Design review of the part built by this model. Coordinates are the model's own, in mm. Give positions to 0.01 mm unless a question says otherwise; leave off trailing zeros. Order: outer loops, then holes, each group sorted by start corner. A loop starts at its lowest first (then second) coordinate and runs counter-clockwise, first axis right, second up. Notation, with made-up numbers: (60.5, 79) -> (118.5, 79) arc R35 ccw to (118.5, 113) -> close; hole circle Ø9 at (51.25, -11.5). An arc over 180 degrees is marked (long way). One line per item, written item: value. Start each with the question number.
1) Consider section C-C (z = 7). State the section outline as (x, y) points (3 decimals), plus the area to 3 significant figures.
2) Consider section A-A (x = 0). State the section outline as (y, z) points (3 decimals).
3) The part is to be moulded in two halves that separate along X. For faces 1 (the face through (9.217, 14.457, 7.357)), 2 (the face through (0, -3, 0)), 3 (the face through (-0.41, -1.86, 7.53)), say which applies: released by +X, released by -X, zero draft, split by the parting line, or undercut.
4) For pin 1 (3 mm diameter, centred on y = -8.5, z = 10, fed in from -X); pin 2 (1.5 mm diameter, centred on x = -8, z = 10.5, fed in from +Y); pin 3 (1.5 mm diameter, centred on x = -13.5, z = 3, fed in from +Y), all flat-tipped, find the tip position at first contact; note any pin that passes through.
5) Wall thickness on line 1 along Y through (x, z) = (0, 6.5) (3 decimals); line 2 along Y through (x, z) = (-0.5, 12); line 3 along X through (y, z) = (-1.5, 4.5): over which ranges is each line inside the solid? List them lowest first. Write a range as from..to.
from build123d import *

# Parameters (mm, degrees)
SKETCH1_R           = 38.1
BOSS_EXTRUDE1_DEPTH = 33.02
FILLET1_R           = 5.08
SCALE1_SCALE        = 0.45
SKETCH3_R           = 1.905
CUT_EXTRUDE1_DEPTH  = 29.437509287


with BuildPart() as part:
    # Sketch1 → Boss-Extrude1 (new body)
    with BuildSketch(Plane.XY):
        Circle(SKETCH1_R)
    extrude(amount=BOSS_EXTRUDE1_DEPTH)

    # Fillet1
    fillet1_edges = [part.edges().sort_by_distance(p)[0] for p in [
        (-38.1, 0, 0),
        (-38.1, 0, 33.02),
    ]]
    fillet(fillet1_edges, radius=FILLET1_R)


with BuildPart() as part_1:
    # Scale1: scaled about (0, 0, 0)
    add(part.part.scale(SCALE1_SCALE))

    # Sketch3 → Cut-Extrude1 (cut, through all)
    with BuildSketch(Plane.XY.offset(14.859)):
        Circle(SKETCH3_R)
    extrude(amount=-CUT_EXTRUDE1_DEPTH, mode=Mode.SUBTRACT)


solid = part_1.part
Checked values:
1. outline: circle Ø34.29 at (0, 0); hole circle Ø3.81 at (0, 0)
1. area: 912 mm^2
2. outline: (-17.145, 2.286) arc R2.286 ccw to (-14.859, 0) -> (-1.905, 0) -> (-1.905, 14.859) -> (-14.859, 14.859) arc R2.286 ccw to (-17.145, 12.573) -> close; (1.905, 0) -> (14.859, 0) arc R2.286 ccw to (17.145, 2.286) -> (17.145, 12.573) arc R2.286 ccw to (14.859, 14.859) -> (1.905, 14.859) -> close
3. face 1: split by the parting line
3. face 2: zero draft
3. face 3: undercut
4. pin 1: stops at x = -15.65
4. pin 2: stops at y = 15.54
4. pin 3: stops at y = 11.46
5. line 1: y = -17.145..-1.905, 1.905..17.145
5. line 2: y = -17.14..-1.84, 1.84..17.14
5. line 3: x = -17.08..-1.17, 1.17..17.08
